Autodesk Inventor part; units mm, degrees
ref_plane "YZ Plane" through (0, 0, 0) normal (1, 0, 0) x (0, 1, 0)
ref_plane "XZ Plane" through (0, 0, 0) normal (0, 1, 0) x (-1, 0, 0)
ref_plane "XY Plane" through (0, 0, 0) normal (0, 0, 1) x (1, 0, 0)
sketch "Esquisse2" plane through (0, 0, 0) normal (0, 1, 0) x (-1, 0, 0)
  line L0 (-7, 113) -> (7, 113)
  line L1 (7, 113) -> (7, -113)
  line L2 (7, -113) -> (-7, -113)
  line L3 (-7, -113) -> (-7, 113)
  line L4 (-7, 113) -> (7, -113) construction
  line L5 (7, 113) -> (-7, -113) construction
  point P0 (0, 0)
  dimension "d0" = 226
  dimension "d1" = 14
extrude "Extrusion1" add sketch "Esquisse2" along normal blind 1
sketch "Esquisse3" plane through (0, 1, 0) normal (0, 1, 0) x (1, 0, 0)
  line L0 (7, 113) -> (-7, 113)
  line L1 (-7, -113) -> (7, -113)
  point P0 (0, 0)
  point P1 (0, -106.5)
  point P2 (0, 108)
  dimension "d4" = 5
  dimension "d14" = 214.5
hole "Perçage1" at (0, 1, 106.5) at (0, 1, -108) direction (0, -1, 0) diameter 4.5 end through all
properties part number "support_lateral" material "Aluminium 6061"
Verification items for the finished model (mm, model axes). Coordinates: 2 decimals unless noted, no trailing zeros. Write each loop counter-clockwise with the first axis right and the second up, starting at its lowest first coordinate (ties: lowest second). Pieces come first, ordered by that corner, then holes. Notation, with made-up numbers: M -34,51.5 L -15,51.5 A20 ccw -15,84.5 Z; hole C -14,45 d9. An arc over 180 degrees is marked long. Use a Markdown table: item, result.
Q1. Sectioned sample at A-A, the plane z = -108. Record the boundary of the cut face in (x, y), plus the area to 3 significant figures.
Reply:
| item | result |
|---|---|
| outline | M -7,0 L -2.25,0 L -2.25,1 L -7,1 Z; M 2.25,0 L 7,0 L 7,1 L 2.25,1 Z |
| area | 9.50 mm² |
Q2. Draft check along Z on faces 1 (the face through (0.86, 0.49, 108.58)), 2 (the face through (0.86, 0.49, -105.92)), 3 (the face through (0, 0, 2)). Enter one of: +Z half, -Z half, draft (parallel to the pull), parting line (faces both ways), or undercut.
Reply:
| item | result |
|---|---|
| face 1 | undercut |
| face 2 | undercut |
| face 3 | draft |
Q3. Go/stop test with flat-tipped pins: P1, Ø5, axis at x = 0, z = -108, coming from the -Y side; P2, Ø3.5, axis at x = 0, z = 106.5, coming from the +Y side. Record where each tip stops, or that it passes through.
Reply:
| item | result |
|---|---|
| P1 | stops at y = 0 |
| P2 | passes through |
Q4. Thickness scan on line 1 (Z direction, x = 0, y = 0.45); line 2 (X direction, y = 0.6, z = 106.5); line 3 (Z direction, x = 1.25, y = 0.6). Record the ranges inside material, lowest first.
Reply:
| item | result |
|---|---|
| line 1 | z = -113 to -110.25, -105.75 to 104.25, 108.75 to 113 |
| line 2 | x = -7 to -2.25, 2.25 to 7 |
| line 3 | z = -113 to -109.87, -106.13 to 104.63, 108.37 to 113 |
